Source: CAD feature listing. Evaluate the final solid. Frame: model axes, mm. A direction names the side the tool comes from. Coordinates: 2 decimals unless noted, no trailing zeros. Loops run counter-clockwise (first coordinate to the right, second up) from the corner with the lowest first, then second, coordinate; pieces in that order, holes last.
from build123d import *

# Parameters (mm, degrees)
SKETCH_2_R          = 1.3
EXTRUDE_1_DEPTH     = 9
SKETCH_3_W          = 30
SKETCH_3_H          = 20.835575778
CUT_EXTRUDE_1_DEPTH = 6
EXTRUDE_START       = -6.7
EXTRUDE_2_DEPTH     = 7
EXTRUDE_3_DEPTH     = 2
EXTRUDE_4_DEPTH     = 2
SKETCH_11_R         = 2.1
EXTRUDE_5_DEPTH     = 7
EXTRUDE_6_DEPTH     = 6
EXTRUDE_7_DEPTH     = 6


with BuildPart() as part:
    # 草图2 → 凸台-拉伸1 (new, symmetric)
    with BuildSketch(Plane.XY):
        Polygon((-11, 11), (11, 11), (15, 7), (15, -11), (-15, -11), (-15, 7), align=None)
        with Locations((-10.3, 5)):
            Circle(SKETCH_2_R, mode=Mode.SUBTRACT)
        with Locations(Location((10.3, 5, 0), (0, 0, 180))):
            Circle(SKETCH_2_R, mode=Mode.SUBTRACT)
    extrude(amount=EXTRUDE_1_DEPTH, both=True)

    # 草图3 → 切除-拉伸1 (cut, symmetric)
    with BuildSketch(Plane.XY):
        with Locations((0, 3.717787889)):
            Rectangle(SKETCH_3_W, SKETCH_3_H)
    extrude(amount=CUT_EXTRUDE_1_DEPTH, both=True, mode=Mode.SUBTRACT)

    # 草图6 → 凸台-拉伸2 (add)
    with BuildSketch(Plane(origin=(0, 0, 0), x_dir=(1, 0, 0), z_dir=(0, 1, 0)).offset(EXTRUDE_START)):
        with BuildLine():
            Line((-20, -15), (20, -15))
            ThreePointArc((20, -15), (27.071067812, -12.071067812), (30, -5))
            Line((30, -5), (30, 23))
            Line((30, 23), (-30, 23))
            Line((-30, 23), (-30, -5))
            ThreePointArc((-30, -5), (-27.071067812, -12.071067812), (-20, -15))
        make_face()
    extrude(amount=-EXTRUDE_2_DEPTH)

    # 草图7 → 凸台-拉伸3 (add)
    with BuildSketch(Plane(origin=(15, 0, 0), x_dir=(0, 0, -1), z_dir=(1, 0, 0))):
        Polygon((-9, 0.3), (-13, -6.7), (-9, -6.7), align=None)
        Polygon((9, -6.7), (9, 0.3), (13, -6.7), align=None)
    extrude(amount=-EXTRUDE_3_DEPTH)

    # 草图10 → 凸台-拉伸4 (add)
    with BuildSketch(Plane.ZY.offset(15)):
        Polygon((-9, 0.15), (-13, -6.7), (-9, -6.7), align=None)
        Polygon((9, -6.7), (9, 0.15), (13, -6.7), align=None)
    extrude(amount=-EXTRUDE_4_DEPTH)

    # 草图11 → 凸台-拉伸5 (add)
    with BuildSketch(Plane.XY.offset(-23)):
        Polygon((-30, -11.7), (30, -11.7), (30, 41.3), (20, 41.3), (20, -3.7), (-20, -3.7), (-20, 41.3), (-30, 41.3), align=None)
        with Locations((-25.5, 33.1)):
            Circle(SKETCH_11_R, mode=Mode.SUBTRACT)
        with Locations((-25.5, 12.1)):
            Circle(SKETCH_11_R, mode=Mode.SUBTRACT)
        with Locations(Location((25.5, 12.1, 0), (0, 0, 180))):
            Circle(SKETCH_11_R, mode=Mode.SUBTRACT)
        with Locations(Location((25.5, 33.1, 0), (0, 0, 180))):
            Circle(SKETCH_11_R, mode=Mode.SUBTRACT)
    extrude(amount=EXTRUDE_5_DEPTH)

    # 草图12 → 凸台-拉伸6 (add)
    with BuildSketch(Plane.ZY.offset(30)):
        Polygon((-4, -6.7), (-16, 5.3), (-16, -6.7), align=None)
    extrude(amount=-EXTRUDE_6_DEPTH)

    # 草图13 → 凸台-拉伸7 (add)
    with BuildSketch(Plane(origin=(30, 0, 0), x_dir=(0, 0, -1), z_dir=(1, 0, 0))):
        Polygon((16, -6.7), (16, 5.3), (4, -6.7), align=None)
    extrude(amount=-EXTRUDE_7_DEPTH)


solid = part.part
Q1. Draft query along X for faces 4 (the flat face through (25, 41.3, -20)), 5 (the flat face through (13, 9, -7)), 6 (the cylindrical face through (-25.773, 14.182, -19.549)). Return one class per face: +X half, -X half, draft (parallel to the pull), parting line (faces both ways), or undercut.
Q2. Access query for faces 1 (the flat face through (27, -0.6, -10.1)), 2 (the flat face through (-13, -5, 10)), 3 (the flat face through (0, -6.7, -1)). Directions: +Z, -Z, +X, -X, +Y, -Y. A direction counts if a zero-diameter tool reaches every point of the face in a straight line with its end or side. Return the directions, or none.
Q3. Section D-D, the plane x = 17.5. Return the cut outline in (y, z), plus the area to 3 significant figures.
Q4. Section C-C, the plane y = 30. Return the cut outline in (x, z).
Q5. Section B-B, the plane z = -20.5. Return the cut outline in (x, y).
Q6. Line query: line 1 along Z through (x, y) = (-1, -4); line 2 along Y through (x, z) = (25.5, -21); line 3 along X through (y, z) = (33, -17). Output: solid intervals per line, ascending.
Q7. Contact query for flat-ended pins moving along their axis: pin 1 Ø2 at (x, z) = (2.5, -18.5) entering from +Y; pin 2 Ø2 at (y, z) = (-1.5, 11.5) entering from -X; pin 3 Ø14 at (x, y) = (2.5, 6.5) entering from -Z; pin 4 Ø5.5 at (x, y) = (25.5, 12.1) entering from +Z. Output: stop coordinate, or through.
Q8. Section A-A, the plane y = 12.1. Return the cut outline in (x, z).
Derived:
1. face 4: draft
1. face 5: +X half
1. face 6: undercut
2. face 1: +Z, +X, +Y
2. face 2: +Z, +Y
2. face 3: +Y
3. outline: (-13.7, -23) - (-3.7, -23) - (-3.7, -16) - (-6.7, -16) - (-6.7, 15) - (-13.7, 15) - close
3. area: 287 mm2
4. outline: (-30, -23) - (-20, -23) - (-20, -16) - (-30, -16) - close; (20, -23) - (30, -23) - (30, -16) - (20, -16) - close
5. outline: (-30, -13.7) - (30, -13.7) - (30, 41.3) - (20, 41.3) - (20, -3.7) - (-20, -3.7) - (-20, 41.3) - (-30, 41.3) - close; hole circle Ø4.2 at (-25.5, 12.1); hole circle Ø4.2 at (-25.5, 33.1); hole circle Ø4.2 at (25.5, 12.1); hole circle Ø4.2 at (25.5, 33.1)
6. line 1: z = -23 to -16, -9 to -6, 6 to 9
6. line 2: y = -13.7 to 10, 14.2 to 31, 35.2 to 41.3
6. line 3: x = -30 to -27.6, -23.4 to -20, 20 to 23.4, 27.6 to 30
7. pin 1: stops at y = -3.7
7. pin 2: passes through
7. pin 3: stops at z = -9
7. pin 4: stops at z = -16
8. outline: (-30, -23) - (-27.6, -23) - (-27.6, -16) - (-30, -16) - close; (-23.4, -23) - (-20, -23) - (-20, -16) - (-23.4, -16) - close; (20, -23) - (23.4, -23) - (23.4, -16) - (20, -16) - close; (27.6, -23) - (30, -23) - (30, -16) - (27.6, -16) - close
